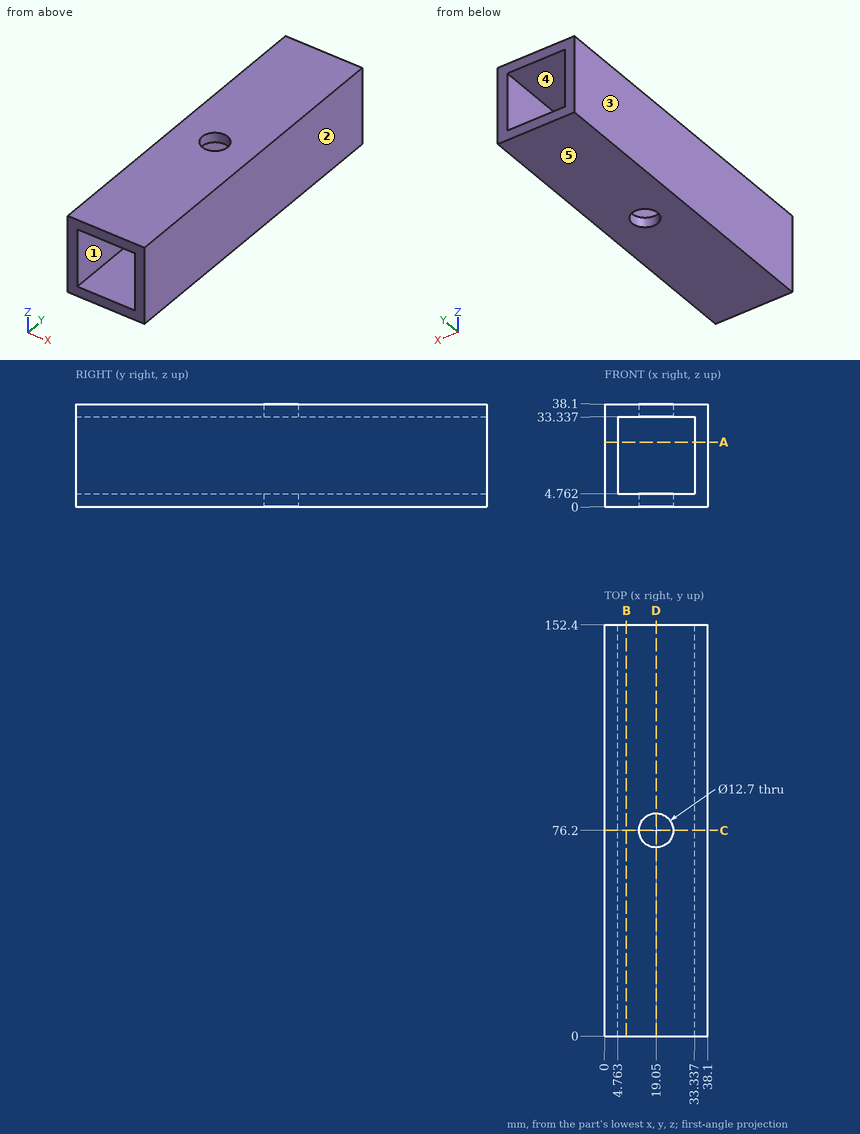
Here's the drawing with two shaded views (mm, measured from the low corner). I have some questions. A direction names the side the tool comes from. Coordinates: 2 decimals unless noted, no trailing zeros. Order: outer loops, then holes, each group sorted by start corner. A loop starts at its lowest first (then second) coordinate and runs counter-clockwise, first axis right, second up. Notation, with made-up numbers: (18, -36.5) - (40, -36.5) arc R30 cw to (40, -3.5) - close; hole circle Ø9 at (22.25, 70.25). An arc over 180 degrees is marked (long way). Answer in a Markdown table with one row per item. Add a question column.
(1) If we section it at A-A, the plane z = 24: Please give me the cut outline in (x, y), then the cut area to 3 significant figures.
(2) If we section it at D-D, the plane x = 19.05: Please give me the cut outline in (y, z).
(3) If we mould it in two halves opening along X, with no side actions, what happens to the marked faces 3, 4 and 5? For each: released by +X, released by -X, zero draft, split by the parting line, or undercut.
(4) If we section it at B-B, the plane x = 8: Please give me the cut outline in (y, z), then the cut area to 3 significant figures.
(5) If we section it at C-C, the plane y = 76.2: Please give me the cut outline in (x, z), then the cut area to 3 significant figures.
(6) I need wall thicknesses on L1, parallel to Z at x = 11.5, y = 119; L2, parallel to Y at x = 19.05, z = 35.9. Which ranges of each line are inside material? Lowest first, please.
(7) On a 3-axis mill with a long thin cutter (end or side, diameter ignored), from which of +Z, -Z, +X, -X, +Y, -Y can I reach the whole of each face in a straight line? I mean the marked faces 1 and 2. Say none if no direction works.
Results are:
| question | item | result |
|---|---|---|
| 1 | outline | (0, 0) - (4.76, 0) - (4.76, 152.4) - (0, 152.4) - close; (33.34, 0) - (38.1, 0) - (38.1, 152.4) - (33.34, 152.4) - close |
| 1 | area | 1,450 mm2 |
| 2 | outline | (0, 0) - (69.85, 0) - (69.85, 4.76) - (0, 4.76) - close; (0, 33.34) - (69.85, 33.34) - (69.85, 38.1) - (0, 38.1) - close; (82.55, 0) - (152.4, 0) - (152.4, 4.76) - (82.55, 4.76) - close; (82.55, 33.34) - (152.4, 33.34) - (152.4, 38.1) - (82.55, 38.1) - close |
| 3 | face 3 | released by -X |
| 3 | face 4 | undercut |
| 3 | face 5 | zero draft |
| 4 | outline | (0, 0) - (152.4, 0) - (152.4, 4.76) - (0, 4.76) - close; (0, 33.34) - (152.4, 33.34) - (152.4, 38.1) - (0, 38.1) - close |
| 4 | area | 1,450 mm2 |
| 5 | outline | (0, 0) - (12.7, 0) - (12.7, 4.76) - (4.76, 4.76) - (4.76, 33.34) - (12.7, 33.34) - (12.7, 38.1) - (0, 38.1) - close; (25.4, 0) - (38.1, 0) - (38.1, 38.1) - (25.4, 38.1) - (25.4, 33.34) - (33.34, 33.34) - (33.34, 4.76) - (25.4, 4.76) - close |
| 5 | area | 514 mm2 |
| 6 | L1 | z = 0 to 4.76, 33.34 to 38.1 |
| 6 | L2 | y = 0 to 69.85, 82.55 to 152.4 |
| 7 | face 1 | +Y, -Y |
| 7 | face 2 | +Z, -Z, +X, +Y, -Y |
